from build123d import *

# Parameters (mm, degrees)
SKETCH_R             = 1
PAD_DEPTH            = 3
SKETCH001_W          = 18.9
SKETCH001_H          = 20
SKETCH001_R          = 1.5
PAD001_DEPTH         = 5
SKETCH002_W          = 2
SKETCH002_H          = 2
PAD002_DEPTH         = 13
SKETCH003_R          = 1.5
PAD003_DEPTH         = 2
SKETCH004_R          = 2
POCKET_DEPTH         = 1
SKETCH005_R          = 3
POCKET001_DEPTH      = 3
POCKET001_DEPTH_BACK = -5


with BuildPart() as part:
    # Sketch (on Face5 of Binder001) → Pad (new body)
    with BuildSketch(Plane(origin=(-16.5, 16.5, 0), x_dir=(0, -1, 0), z_dir=(0, 0, 1))):
        with BuildLine():
            Line((-20.2, 25.2), (20.2, 25.2))
            Line((20.2, 25.2), (20.2, 20.2))
            Line((20.2, 20.2), (20.2, -16.25))
            ThreePointArc((12.3, -16.25), (16.25, -20.2), (20.2, -16.25))
            Line((12.3, -12.448293), (12.3, -16.25))
            ThreePointArc((12.3, -12.448293), (0, 17.5), (-12.3, -12.448293))
            Line((-12.3, -16.25), (-12.3, -12.448293))
            ThreePointArc((-20.2, -16.25), (-16.25, -20.2), (-12.3, -16.25))
            Line((-20.2, 20.2), (-20.2, -16.25))
            Line((-20.2, 20.2), (-20.2, 25.2))
        make_face()
        with Locations((-16.25, 16.25)):
            Circle(SKETCH_R, mode=Mode.SUBTRACT)
        with Locations((16.25, 16.25)):
            Circle(SKETCH_R, mode=Mode.SUBTRACT)
        with Locations((16.25, -16.25)):
            Circle(SKETCH_R, mode=Mode.SUBTRACT)
        with Locations((-16.25, -16.25)):
            Circle(SKETCH_R, mode=Mode.SUBTRACT)
    extrude(amount=PAD_DEPTH)

    # Sketch001 (on Face4 of Pad) → Pad001 (join)
    with BuildSketch(Plane(origin=(8.7, 16.5, -29.5), x_dir=(0, 1, 0), z_dir=(1, 0, 0))):
        with Locations((0, 19.5)):
            Rectangle(SKETCH001_W, SKETCH001_H)
        with Locations((-5, 27)):
            Circle(SKETCH001_R, mode=Mode.SUBTRACT)
        with Locations((5, 27)):
            Circle(SKETCH001_R, mode=Mode.SUBTRACT)
        with Locations((-5, 12)):
            Circle(SKETCH001_R, mode=Mode.SUBTRACT)
        with Locations((5, 12)):
            Circle(SKETCH001_R, mode=Mode.SUBTRACT)
    extrude(amount=-PAD001_DEPTH)

    # Sketch002 (on Face10 of Pad001) → Pad002 (join)
    with BuildSketch(Plane(origin=(3.7, 16.5, -29.5), x_dir=(0, -1, 0), z_dir=(-1, 0, 0))):
        with Locations((-8.45, 8.5)):
            Rectangle(SKETCH002_W, SKETCH002_H)
    extrude(amount=-PAD002_DEPTH)

    # Sketch003 (on Face30 of Pad002) → Pad003 (join)
    with BuildSketch(Plane(origin=(16.7, 16.5, -29.5), x_dir=(0, 1, 0), z_dir=(1, 0, 0))):
        Polygon((4.45, 2.35), (9.45, 2.35), (9.45, 9.5), (7.45, 9.5), (7.45, 7.5), (4.45, 6.35), align=None)
        with Locations((6.95, 4.85)):
            Circle(SKETCH003_R, mode=Mode.SUBTRACT)
    extrude(amount=-PAD003_DEPTH)

    # Sketch004 (on Face35 of Pad003) → Pocket (cut)
    with BuildSketch(Plane(origin=(14.7, 16.5, -29.5), x_dir=(0, -1, 0), z_dir=(-1, 0, 0))):
        with Locations((-6.95, 4.85)):
            Circle(SKETCH004_R)
    extrude(amount=-POCKET_DEPTH, mode=Mode.SUBTRACT)

    # Sketch005 (on Face10 of Pocket) → Pocket001 (cut, two sides)
    with BuildSketch(Plane(origin=(3.7, 16.5, -29.5), x_dir=(0, -1, 0), z_dir=(-1, 0, 0))) as pocket001_sk:
        with Locations((-5, 27)):
            Circle(SKETCH005_R)
        with Locations((5, 27)):
            Circle(SKETCH005_R)
        with BuildLine():
            ThreePointArc((-2, 12.000001), (-5, 15), (-8, 12.000001))
            Line((-8, 7.5), (-8, 12.000001))
            Line((-2, 7.5), (-8, 7.5))
            Line((-2, 12.000001), (-2, 7.5))
        make_face()
        with BuildLine():
            ThreePointArc((8, 11.999976), (5, 15), (2, 11.999976))
            Line((2, 11.999976), (2, 9.5))
            Line((2, 9.5), (8, 9.5))
            Line((8, 9.5), (8, 11.999976))
        make_face()
    extrude(amount=-POCKET001_DEPTH, mode=Mode.SUBTRACT)
    extrude(pocket001_sk.sketch, amount=-POCKET001_DEPTH_BACK, mode=Mode.SUBTRACT)


with BuildPart() as part_1:
    # Body placement: moved
    add(part.part.moved(Location((0, 0, -4))))


solid = part_1.part
Verification items for the finished model (mm, model axes). A direction names the side the tool comes from. Coordinates: 2 decimals unless noted, no trailing zeros. Write each loop counter-clockwise with the first axis right and the second up, starting at its lowest first coordinate (ties: lowest second). Pieces come first, ordered by that corner, then holes. Notation, with made-up numbers: (12, 39.25) - (17, 39.25) arc R21 cw to (17, 54.25) - close; hole circle Ø1 at (89.25, 17.5). An arc over 180 degrees is marked (long way). Answer as a JSON object with one key per item and string values.
(1) Cross-section at A-A on z = -6.5. Record the cut outline in (x, y).
Report:
{"outline": "(3.7, 7.05) - (8.7, 7.05) - (8.7, 10) - (6.7, 10) - (6.7, 8.5) - (3.7, 8.5) - close; (3.7, 14.5) - (6.7, 14.5) - (6.7, 13) - (8.7, 13) - (8.7, 20) - (6.7, 20) - (6.7, 18.5) - (3.7, 18.5) - close; (3.7, 24.5) - (6.7, 24.5) - (6.7, 23) - (8.7, 23) - (8.7, 25.95) - (3.7, 25.95) - close"}
(2) Cross-section at B-B on x = 6. Record the cut outline in (y, z), plus the area to 3 significant figures.
Report:
{"outline": "(-3.7, -4) - (7.05, -4) - (7.05, -24) - (8.5, -24) - (8.5, -21.5) arc R3 cw to (14.5, -21.5) - (14.5, -24) - (18.5, -24) - (18.5, -21.5) arc R3 cw to (24.5, -21.5) - (24.5, -26) - (25.95, -26) - (25.95, -4) - (36.7, -4) - (36.7, -1) - (-3.7, -1) - close; hole circle Ø6 at (11.5, -6.5); hole circle Ø6 at (21.5, -6.5)", "area": "387 mm^2"}
(3) Mould release check, pull along X, two halves, no side actions. Record for faces 1 (the flat face through (8.7, 17, -10)), 2 (the cylindrical face through (-36.7, 32.8, -2.5)), 3 (the flat face through (-31, 4.2, -3)), 4 (the cylindrical face through (-31.76, 0.38, -2.52)): pulls with the +X half, pulls with the -X half, needs draft (parallel to the pull), parting line crosses it, or undercut.
Report:
{"face 1": "pulls with the +X half", "face 2": "pulls with the -X half", "face 3": "needs draft", "face 4": "undercut"}
(4) Tool access check on faces 5 (the flat face through (5, 24.5, -24)), 6 (the flat face through (9, 25, -26)), 7 (the cylindrical face through (-0.86, 1.04, -2.52)), 8 (the flat face through (7, 15, -24)). Record the directions out of +Z, -Z, +X, -X, +Y, -Y that give a thin tool (end or side, any length) a straight path to the whole face; none if there is none.
Report:
{"face 5": "-Z, -X", "face 6": "-Z, -X, +Y, -Y", "face 7": "+Z, -Z", "face 8": "-Z, +X, -X, -Y"}
(5) Cross-section at C-C on x = -31. Record the cut outline in (y, z).
Report:
{"outline": "(-3.7, -4) - (4.2, -4) - (4.2, -1) - (-3.7, -1) - close; (28.8, -4) - (36.7, -4) - (36.7, -1) - (28.8, -1) - close"}
(6) Gauge pin test, flat ends, axial feed: pin 1 Ø2 at (x, y) = (12, 25) entering from +Z; pin 2 Ø1.6 at (x, z) = (15.5, -30) entering from -Y; pin 3 Ø12 at (y, z) = (30.5, -10.5) entering from -X. Record the tip position at first contact, or that the pin passes through.
Report:
{"pin 1": "z = -24", "pin 2": "y = 20.95", "pin 3": "x = 3.7"}
(7) Cross-section at D-D on y = 0.25. Record the cut outline in (x, z).
Report:
{"outline": "(-36.7, -4) - (-33.75, -4) - (-33.75, -1) - (-36.7, -1) - close; (-31.75, -4) - (-23, -4) - (-23, -1) - (-31.75, -1) - close; (-10, -4) - (-1.25, -4) - (-1.25, -1) - (-10, -1) - close; (0.75, -4) - (8.7, -4) - (8.7, -1) - (0.75, -1) - close"}
(8) Thickness scan on line 1 along Z through (x, y) = (8.1, 11.5); line 2 along Y through (x, z) = (-16, -2); line 3 along Z through (x, y) = (3, 2.5). Record the ranges inside material, lowest first.
Report:
{"line 1": "-24 to -23, -20 to -8, -5 to -1", "line 2": "-3.7 to -0.99, 33.99 to 36.7", "line 3": "-4 to -1"}
